For this review, take the finished solid that the model builds, in its own axes (mm). Face numbers are marked on the shaded views. Round coordinates to 2 decimals unless told otherwise and drop trailing zeros. Write each loop counter-clockwise with the first axis right and the second up, starting at its lowest first coordinate (ties: lowest second). Pieces come first, ordered by that corner, then holes. Notation, with made-up numbers: (76.5, -6.5) -> (117.5, -6.5) arc R16 ccw to (117.5, 17.5) -> close; hole circle Ø1 at (78.25, 59). An arc over 180 degrees is marked (long way). Write item = value, one per line. Start each with the question number.
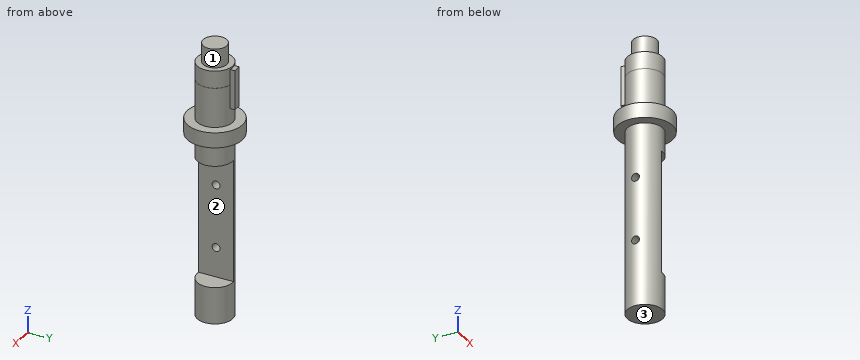
```python
from build123d import *

# Parameters (mm, degrees)
SKETCH2_R               = 28.15
BOSS_EXTRUDE1_DEPTH     = 62.5
BOSS_EXTRUDE2_START     = 25
BOSS_EXTRUDE2_DEPTH     = 62.5
SKETCH5_W               = 31.1
SKETCH5_H               = 193.8
CUT_EXTRUDE1_DEPTH      = 44.6
CUT_EXTRUDE1_DEPTH_BACK = 44.6
SKETCH6_R               = 6.25
CUT_EXTRUDE2_DEPTH      = 41.5


with BuildPart() as part:
    # Sketch1 → Revolve1 (revolve)
    with BuildSketch(Plane(origin=(0, 0, 0), x_dir=(1, 0, 0), z_dir=(0, 1, 0))):
        Polygon((0, 0), (28, 0), (28, -290), (43.6, -290), (43.6, -314), (28, -314), (28, -403.8), (18.75, -403.8), (18.75, -433.8), (0, -433.8), align=None)
    revolve(axis=Axis((0, 0, 0), (0, 0, 1)))

    # Sketch2 → Boss-Extrude1 (add)
    with BuildSketch(Plane.XY.offset(314)):
        Circle(SKETCH2_R)
    extrude(amount=BOSS_EXTRUDE1_DEPTH)

    # Sketch3 → Boss-Extrude2 (add)
    with BuildSketch(Plane.XY.offset(314).offset(BOSS_EXTRUDE2_START)):
        with BuildLine():
            Line((-6.3, 35), (6.3, 35))
            Line((6.3, 35), (6.3, 27.435970914))
            ThreePointArc((6.3, 27.435970914), (0, 28.15), (-6.3, 27.435970914))
            Line((-6.3, 27.435970914), (-6.3, 35))
        make_face()
    extrude(amount=BOSS_EXTRUDE2_DEPTH)

    # Sketch5 → Cut-Extrude1 (cut, two sides)
    with BuildSketch(Plane(origin=(0, 0, 0), x_dir=(1, 0, 0), z_dir=(0, 1, 0))) as cut_extrude1_sk:
        with Locations((12.45, -154.9)):
            Rectangle(SKETCH5_W, SKETCH5_H)
    extrude(amount=CUT_EXTRUDE1_DEPTH, mode=Mode.SUBTRACT)
    extrude(cut_extrude1_sk.sketch, amount=-CUT_EXTRUDE1_DEPTH_BACK, mode=Mode.SUBTRACT)

    # Sketch6 → Cut-Extrude2 (cut, through all)
    with BuildSketch(Plane(origin=(-3.1, 0, 0), x_dir=(0, 0, -1), z_dir=(1, 0, 0))):
        with Locations((-204.9, 0)):
            Circle(SKETCH6_R)
        with Locations((-104.9, 0)):
            Circle(SKETCH6_R)
    extrude(amount=-CUT_EXTRUDE2_DEPTH, mode=Mode.SUBTRACT)


solid = part.part
```
1. Consider section D-D, the plane x = -36.5. Give the boundary of the cut face in (y, z).
2. Draft analysis for pull direction Z (two halves, no side actions). For the marked faces 1, 2 and 3, state which applies: +Z half, -Z half, draft (parallel to the pull), parting line (faces both ways), or undercut.
3. Consider section C-C, the plane z = 280. Give the boundary of the cut face in (x, y).
4. Consider section A-A, the plane y = 0. Give the number of separate pieces and of enclosed holes in the cut face, then the cut area to 3 significant figures.
5. Consider section B-B, the plane z = 204.9. Give the boundary of the cut face in (x, y).
6. Wall thickness on L1, parallel to Z at x = -15, y = 0; L2, parallel to Z at x = 4.5, y = 19; L3, parallel to Z at x = 16.5, y = -2.5: over which ranges is each line inside the solid? List them lowest first. Write a range as from..to.
7. Clearance check with flat-ended pins moving along their axes: pin 1 Ø8.5 at (y, z) = (29.5, 377.5) entering from +X; pin 2 Ø1 at (x, y) = (-6, 31.5) entering from -Z; pin 3 Ø16.5 at (y, z) = (5.5, 124.5) entering from +X. State where each tip first meets the part, or that it passes through.
Outcome:
q1.outline = (-23.85, 290) -> (23.85, 290) -> (23.85, 314) -> (-23.85, 314) -> close
q2.face_1 = draft
q2.face_2 = undercut
q2.face_3 = -Z half
q3.outline = circle Ø56 at (0, 0)
q4.separate_pieces = 3
q4.enclosed_holes = 0
q4.area = 17,900 mm2
q5.outline = (-27.29, -6.25) arc R28 ccw to (-3.1, -27.83) -> (-3.1, -6.25) -> close; (-27.29, 6.25) -> (-3.1, 6.25) -> (-3.1, 27.83) arc R28 ccw to start
q6.L1 = 0..98.65, 111.15..198.65, 211.15..433.8
q6.L2 = 0..58, 251.8..403.8
q6.L3 = 0..58, 251.8..433.8
q7.pin_1 = 12.2
q7.pin_2 = 290
q7.pin_3 = -3.1
